Geometry check sheet. Reference: drawing and pictorial views, mm from the part's lowest x, y, z. A direction names the side the tool comes from. Give positions to 0.01 mm unless a question says otherwise; leave off trailing zeros. Loops run counter-clockwise (first coordinate to the right, second up) from the corner with the lowest first, then second, coordinate; pieces in that order, holes last. Notation, with made-up numbers: (-2.5, -32) - (12.5, -32) arc R11 ccw to (12.5, -11) - close; hole circle Ø4 at (-21.5, 43). An arc over 180 degrees is marked (long way). Put each result on its own line as item: value. Start each with the question number.
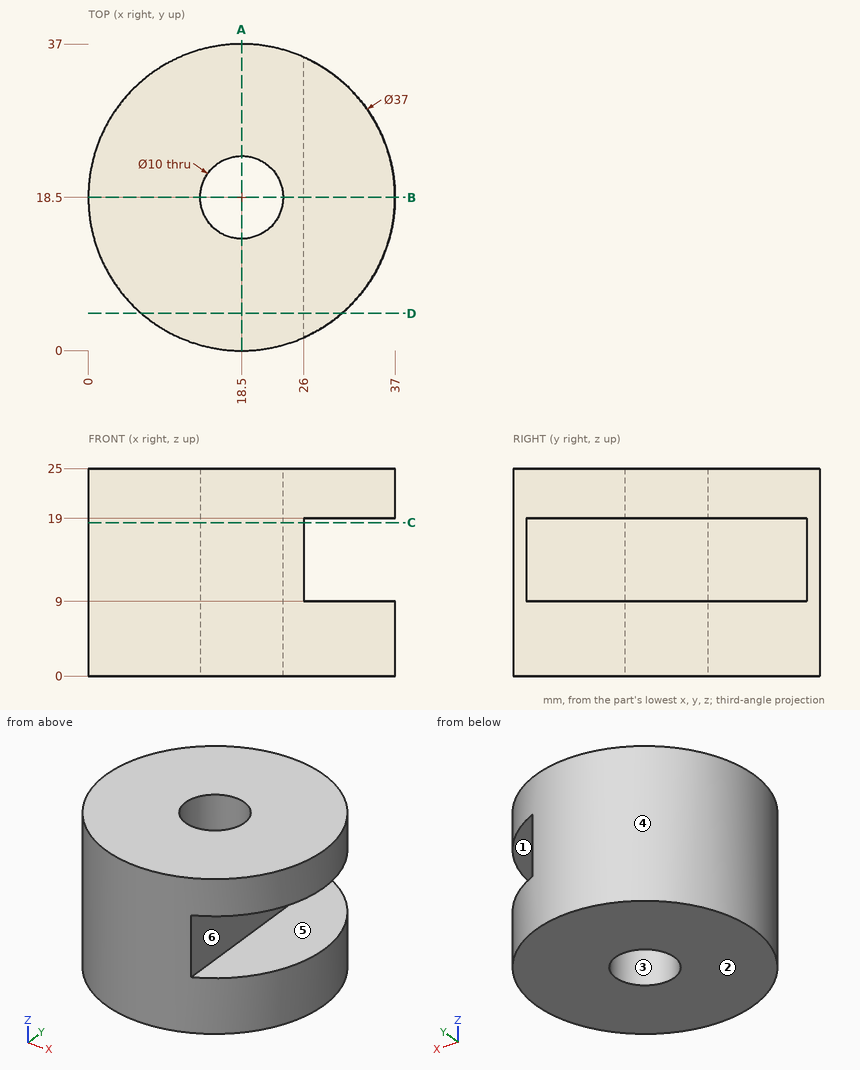
1) Section check C-C, the plane z = 18.5. Enter the section's corners in (x, y), plus the area to 3 significant figures.
2) Section check D-D, the plane y = 4.5. Enter the section's corners in (x, z).
3) Depth check by flat-ended pin: P1, Ø1, axis at y = 7, z = 3.5, coming from the +X side; P2, Ø4, axis at x = 30.5, z = 5, coming from the +Y side; P3, Ø5, axis at y = 13, z = 15.5, coming from the +X side. Enter the tip coordinate at first touch or a pass-through.
4) Section check A-A, the plane x = 18.5. Enter the section's corners in (y, z).
5) Draft check along X on the marked faces 3, 4, 5 and 6. Enter one of: pulls with the +X half, pulls with the -X half, needs draft (parallel to the pull), parting line crosses it, or undercut.
6) Set-up check for the marked faces 1 and 2: record each of +Z, -Z, +X, -X, +Y, -Y from which the full face is reachable in a straight line by a thin tool's end or side.
7) Section check B-B, the plane y = 18.5. Enter the section's corners in (x, z), plus the area to 3 significant figures.
8) Scan lines: line 1 along Z through (x, y) = (30, 19); line 2 along Y through (x, z) = (18.5, 10.75); line 3 along Y through (x, z) = (22.5, 15). Record each from-to range of solid material in increasing order. Write a range as from..to.
Results are:
1. outline: (26, 1.59) - (26, 35.41) arc R18.5 ccw (long way) to start; hole circle Ø10 at (18.5, 18.5)
1. area: 729 mm2
2. outline: (6.41, 0) - (30.59, 0) - (30.59, 9) - (26, 9) - (26, 19) - (30.59, 19) - (30.59, 25) - (6.41, 25) - close
3. P1: stops at x = 33.37
3. P2: stops at y = 34.06
3. P3: stops at x = 26
4. outline: (0, 0) - (13.5, 0) - (13.5, 25) - (0, 25) - close; (23.5, 0) - (37, 0) - (37, 25) - (23.5, 25) - close
5. face 3: undercut
5. face 4: parting line crosses it
5. face 5: needs draft
5. face 6: pulls with the +X half
6. face 1: +X, +Y, -Y
6. face 2: -Z, +X, -X, +Y, -Y
7. outline: (0, 0) - (13.5, 0) - (13.5, 25) - (0, 25) - close; (23.5, 0) - (37, 0) - (37, 9) - (26, 9) - (26, 19) - (37, 19) - (37, 25) - (23.5, 25) - close
7. area: 565 mm2
8. line 1: z = 0..9, 19..25
8. line 2: y = 0..13.5, 23.5..37
8. line 3: y = 0.44..15.5, 21.5..36.56
